from build123d import *

# Parameters (mm, degrees)
BOSS_EXTRUDE1_DEPTH = 1.5875
CUT_EXTRUDE1_DEPTH  = 379.865331816
CUT_EXTRUDE2_DEPTH  = 379.865331816
FILLET1_R           = 12.7
FILLET2_R           = 5.08


with BuildPart() as part:
    # Sketch1 → Boss-Extrude1 (new body)
    with BuildSketch(Plane(origin=(0, 0, 0), x_dir=(1, 0, 0), z_dir=(0, 1, 0))):
        Polygon((-207.536668491, 316.962065124), (-186.581668491, 316.962065124), (-185.030654327, 312.392094548), (-164.710654327, 312.392094548), (50.8, 4.826), (0, 4.826), (0, 0), (-50.8, 0), (-50.8, 4.826), (-101.6, 4.826), align=None)
    extrude(amount=BOSS_EXTRUDE1_DEPTH)

    # Sketch2 → Cut-Extrude1 (cut, through all)
    with BuildSketch(Plane(origin=(0, 1.5875, 0), x_dir=(1, 0, 0), z_dir=(0, 1, 0))):
        Polygon((-103.511728228, 158.75), (-103.511728228, 152.654), (-151.771728228, 152.654), (-153.840665475, 158.75), align=None)
    extrude(amount=-CUT_EXTRUDE1_DEPTH, mode=Mode.SUBTRACT)

    # Sketch3 → Cut-Extrude2 (cut, through all)
    with BuildSketch(Plane(origin=(0, 1.5875, 0), x_dir=(1, 0, 0), z_dir=(0, 1, 0))):
        Polygon((-116.328139028, 127.254), (-83.397554521, 30.226), (1.987487188, 30.226), (-65.999745926, 127.254), align=None)
        Polygon((-167.286096734, 261.592094548), (-145.313109394, 196.85), (-108.562496075, 196.85), (-153.927090567, 261.592094548), align=None)
    extrude(amount=-CUT_EXTRUDE2_DEPTH, mode=Mode.SUBTRACT)

    # Fillet1
    fillet1_edges = [part.edges().sort_by_distance(p)[0] for p in [
        (-116.328139028, 0.79375, -127.254),
        (-65.999745926, 0.79375, -127.254),
        (1.987487188, 0.79375, -30.226),
        (-83.397554521, 0.79375, -30.226),
    ]]
    fillet(fillet1_edges, radius=FILLET1_R)

    # Fillet2
    fillet2_edges = [part.edges().sort_by_distance(p)[0] for p in [
        (-167.286096734, 0.79375, -261.592094548),
        (-153.927090567, 0.79375, -261.592094548),
        (-108.562496075, 0.79375, -196.85),
        (-145.313109394, 0.79375, -196.85),
    ]]
    fillet(fillet2_edges, radius=FILLET2_R)


solid = part.part
Check sheet for the modelled part. Datum: model origin and axes. Units: mm. A direction names the side the tool comes from. Coordinates: 2 decimals unless noted, no trailing zeros. Write each loop counter-clockwise with the first axis right and the second up, starting at its lowest first coordinate (ties: lowest second). Pieces come first, ordered by that corner, then holes. Notation, with made-up numbers: M 36.5,-1 L 56.5,-1 A16 ccw 56.5,24 Z; hole C -5.5,-2.5 d1. An arc over 180 degrees is marked long. Answer as CSV lines item,"result".
Q1. Cross-section at A-A (z = -72). Record the boundary of the cut face in (x, y), then the cut area to 3 significant figures.
Check result:
outline,"M -124.4,0 L -97.58,0 L -97.58,1.59 L -124.4,1.59 Z; M -27.28,0 L 3.73,0 L 3.73,1.59 L -27.28,1.59 Z"
area,"91.8 mm^2"
Q2. Set-up check for faces 1 (the face through (-97, 1.588, -147)), 2 (the face through (-155.875, 0.805, -227.97)): record each of +Z, -Z, +X, -X, +Y, -Y from which the full face is reachable in a straight line by a thin tool's end or side.
Check result:
face 1,"+Z, -Z, +X, -X, +Y"
face 2,"+Y, -Y"
Q3. Cross-section at B-B (y = 0.6). Count the separate pieces of the cut face and the enclosed holes in it, then the cut area to 3 significant figures.
Check result:
separate pieces,"1"
enclosed holes,"2"
area,"21,900 mm^2"
Q4. Material ranges on probe 1 along X at (y, z) = (0.2, -253); probe 2 along Z at (x, y) = (-82, 0.85); probe 3 along X at (y, z) = (1.4, -72), recorded low to high. Write a range as from..to.
Check result:
probe 1,"-185.83..-164.37, -147.91..-123.09"
probe 2,"-194.35..-127.25, -32.83..-4.83"
probe 3,"-124.4..-97.58, -27.28..3.73"
Q5. Cross-section at D-D (x = -91). Record the boundary of the cut face in (y, z).
Check result:
outline,"M 0,-207.2 L 1.59,-207.2 L 1.59,-127.25 L 0,-127.25 Z; M 0,-52.63 L 1.59,-52.63 L 1.59,-4.83 L 0,-4.83 Z"
Q6. Mould release check, pull along X, two halves, no side actions. Record for faces 3 (the face through (-180.313, 0.783, -236.749)), 4 (the face through (-97, 0, -147)), 5 (the face through (-133.02, 0.805, -231.754)): released by +X, released by -X, zero draft, split by the parting line, or undercut.
Check result:
face 3,"released by -X"
face 4,"zero draft"
face 5,"undercut"
Q7. Go/stop test with flat-tipped pins: pin 1 (0.5 mm diameter, centred on y = 0.5, z = -2, fed in from -X); pin 2 (0.8 mm diameter, centred on x = -48, y = 1, fed in from -Z); pin 3 (0.8 mm diameter, centred on x = -79.5, y = 1, fed in from +Z). Record where each tip stops, or that it passes through.
Check result:
pin 1,"x = -50.8"
pin 2,"z = -146.4"
pin 3,"z = -4.83"
Q8. Cross-section at C-C (x = -124). Record the boundary of the cut face in (y, z), then the cut area to 3 significant figures.
Check result:
outline,"M 0,-254.29 L 1.59,-254.29 L 1.59,-218.88 L 0,-218.88 Z; M 0,-196.85 L 1.59,-196.85 L 1.59,-158.75 L 0,-158.75 Z; M 0,-152.65 L 1.59,-152.65 L 1.59,-70.83 L 0,-70.83 Z"
area,"247 mm^2"
